Can you work these out from the model? Positions are in its coordinate system, mm. Face numbers are marked on the shaded views. Give positions to 0.01 mm unless a question says otherwise; leave off trailing zeros. Loops run counter-clockwise (first coordinate to the right, second up) from the corner with the lowest first, then second, coordinate; pieces in that order, holes last. Notation, with made-up numbers: M 45,-9.75 L 63,-9.75 A8 cw 63,1.25 Z; hole C 73,27 d11. An arc over 180 degrees is marked long. Put each result on its own line as item: value. Start each with the question number.
1) If we mould it in two halves opening along Y, with no side actions, what happens to the marked faces 1, 2 and 3? For each: +Y half, -Y half, draft (parallel to the pull), parting line (faces both ways), or undercut.
2) Imagine slicing it at D-D (z = 1.7). Write out the boundary of the cut face in (x, y) (3 decimals), then the cut area to 3 significant figures.
3) Imagine slicing it at B-B (x = 26). Write out the boundary of the cut face in (y, z) (3 decimals).
4) Please list where these lines run through material, in increasing order: line 1 along Y through (x, z) = (5.08, 1.1); line 2 along Y through (x, z) = (15.5, 2.7); line 3 along X through (y, z) = (4, 2.35). Write a range as from..to.
5) Imagine slicing it at A-A (y = 10.16). Write out the boundary of the cut face in (x, z) (3 decimals).
6) Imagine slicing it at C-C (x = 5.08). Write out the boundary of the cut face in (y, z) (3 decimals).
from build123d import *

# Parameters (mm, degrees)
SKETCH1_R           = 2.15265
SKETCH1_W           = 39.624
SKETCH1_H           = 4.572
BOSS_EXTRUDE1_DEPTH = 3.175


with BuildPart() as part:
    # Sketch1 → Boss-Extrude1 (new body)
    with BuildSketch(Plane.XY):
        with BuildLine():
            Line((0, 0), (0, 20.32))
            Line((0, 20.32), (44.45, 20.32))
            ThreePointArc((44.45, 20.32), (54.61, 10.16), (44.45, 0))
            Line((44.45, 0), (0, 0))
        make_face()
        with Locations((5.08, 15.875)):
            Circle(SKETCH1_R, mode=Mode.SUBTRACT)
        with Locations(Location((5.08, 4.445, 0), (0, 0, 180))):
            Circle(SKETCH1_R, mode=Mode.SUBTRACT)
        with Locations((29.972, 10.16)):
            Rectangle(SKETCH1_W, SKETCH1_H, mode=Mode.SUBTRACT)
    extrude(amount=BOSS_EXTRUDE1_DEPTH)


solid = part.part
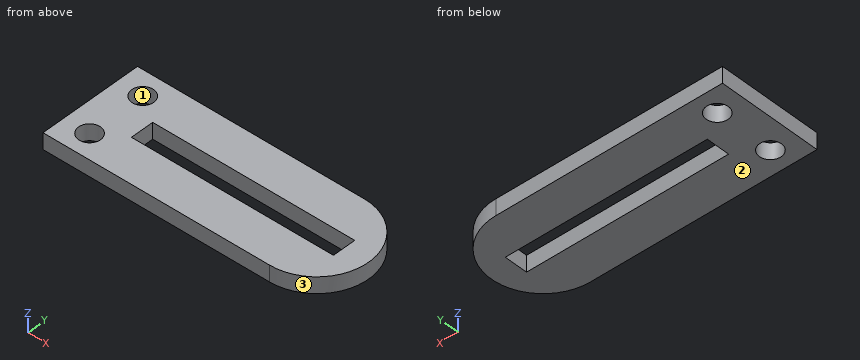
Recorded:
1. face 1: undercut
1. face 2: draft
1. face 3: parting line
2. outline: M 0,0 L 44.45,0 A10.16 ccw 44.45,20.32 L 0,20.32 Z; hole C 5.08,4.445 d4.305; hole C 5.08,15.875 d4.305; hole M 10.16,7.874 L 49.784,7.874 L 49.784,12.446 L 10.16,12.446 Z
2. area: 855 mm²
3. outline: M 0,0 L 7.874,0 L 7.874,3.175 L 0,3.175 Z; M 12.446,0 L 20.32,0 L 20.32,3.175 L 12.446,3.175 Z
4. line 1: 0..2.29, 6.6..13.72, 18.03..20.32
4. line 2: 0..7.87, 12.45..20.32
4. line 3: 0..2.97, 7.19..52.53
5. outline: M 0,0 L 10.16,0 L 10.16,3.175 L 0,3.175 Z; M 49.784,0 L 54.61,0 L 54.61,3.175 L 49.784,3.175 Z
6. outline: M 0,0 L 2.292,0 L 2.292,3.175 L 0,3.175 Z; M 6.598,0 L 13.722,0 L 13.722,3.175 L 6.598,3.175 Z; M 18.028,0 L 20.32,0 L 20.32,3.175 L 18.028,3.175 Z
